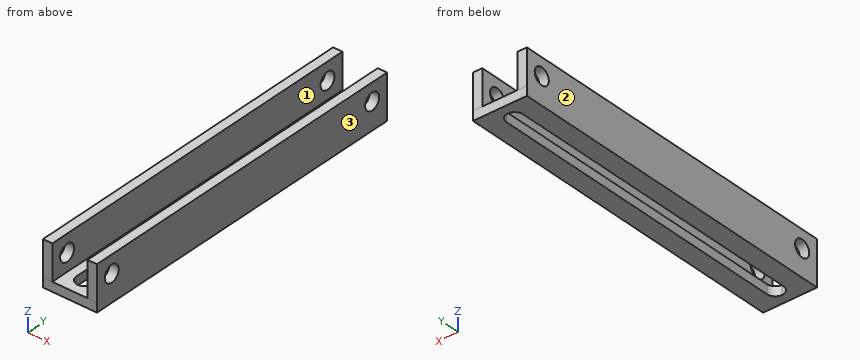
from build123d import *

# Parameters (mm, degrees)
PAD_DEPTH               = 3
SKETCH001_W             = 55.7
SKETCH001_H             = 14.4
SKETCH001_R             = 2.7
PAD001_DEPTH            = 3
PAD_MIRRORED_2_DEPTH    = 3
SKETCH001_MIRRORED_2_W  = 55.7
SKETCH001_MIRRORED_2_H  = 14.4
SKETCH001_MIRRORED_2_R  = 2.7
PAD001_MIRRORED_2_DEPTH = 3


with BuildPart() as part:
    # Sketch → Pad (new body)
    with BuildSketch(Plane.XY):
        with BuildLine():
            ThreePointArc((2.7, 50), (1.909196, 51.909202), (0, 52.700021))
            Line((0, 52.700021), (0, 55.700021))
            Line((0, 55.700021), (8.7, 55.700021))
            Line((8.7, 55.700021), (8.7, 0))
            Line((8.7, 0), (2.7, 0))
            Line((2.7, 0), (2.7, 50))
        make_face()
    pad = extrude(amount=PAD_DEPTH)

    # Sketch001 → Pad001 (join)
    with BuildSketch(Plane.YZ.offset(8.7)):
        with Locations((27.85, 7.2)):
            Rectangle(SKETCH001_W, SKETCH001_H)
        with Locations((50, 8.7)):
            Circle(SKETCH001_R, mode=Mode.SUBTRACT)
    pad001 = extrude(amount=-PAD001_DEPTH)

    # Sketch Mirrored 2 → Pad Mirrored 2 (add)
    with BuildSketch(Plane(origin=(0, 0, 0), x_dir=(-1, 0, 0), z_dir=(0, 0, -1))):
        with BuildLine():
            ThreePointArc((2.7, 50), (1.909196, 51.909202), (0, 52.700021))
            Line((0, 52.700021), (0, 55.700021))
            Line((0, 55.700021), (8.7, 55.700021))
            Line((8.7, 55.700021), (8.7, 0))
            Line((8.7, 0), (2.7, 0))
            Line((2.7, 0), (2.7, 50))
        make_face()
    pad_mirrored_2 = extrude(amount=-PAD_MIRRORED_2_DEPTH)

    # Sketch001 Mirrored 2 → Pad001 Mirrored 2 (add)
    with BuildSketch(Plane.YZ.offset(-8.7)):
        with Locations((27.85, 7.2)):
            Rectangle(SKETCH001_MIRRORED_2_W, SKETCH001_MIRRORED_2_H)
        with Locations((50, 8.7)):
            Circle(SKETCH001_MIRRORED_2_R, mode=Mode.SUBTRACT)
    pad001_mirrored_2 = extrude(amount=PAD001_MIRRORED_2_DEPTH)

    # Mirrored001: Pad, Pad001, Pad Mirrored 2, Pad001 Mirrored 2 across Sketch H_Axis
    add(pad.mirror(Plane.ZX))
    add(pad001.mirror(Plane.ZX))
    add(pad_mirrored_2.mirror(Plane.ZX))
    add(pad001_mirrored_2.mirror(Plane.ZX))


solid = part.part
The model under review builds one solid part; all positions refer to its coordinate system, in mm. Face numbers are marked on the shaded views. Round coordinates to 2 decimals unless told otherwise and drop trailing zeros. Loops run counter-clockwise (first coordinate to the right, second up) from the corner with the lowest first, then second, coordinate; pieces in that order, holes last. Notation, with made-up numbers: (-10.5, 40.5) -> (18.5, 40.5) arc R28 cw to (18.5, 64.5) -> close; hole circle Ø7 at (-23, 5). An arc over 180 degrees is marked (long way). One line per question, with ' | ' between items. Start each with the question number.
Item 1: Draft analysis for pull direction X (two halves, no side actions). For the marked faces 1, 2 and 3, state which applies: +X half, -X half, draft (parallel to the pull), parting line (faces both ways), or undercut.
Item 2: Wall thickness on line 1 along Z through (x, y) = (6.65, 50); line 2 along X through (y, z) = (-16, 5); line 3 along Y through (x, z) = (-6.25, 11): over which ranges is each line inside the solid? List them lowest first. Write a range as [from, to].
Item 3: Add section A-A, the plane z = 8.7. Write out the cut boundary in (x, y), then the cut area to 3 significant figures.
Item 4: Add section B-B, the plane y = -8.5. Write out the cut boundary in (x, z).
Item 5: Add section C-C, the plane x = 1.25. Write out the cut boundary in (y, z).
Return value:
1) face 1: undercut | face 2: -X half | face 3: +X half
2) line 1: z = [0, 6], [11.4, 14.4] | line 2: x = [-8.7, -5.7], [5.7, 8.7] | line 3: y = [-55.7, -51.41], [-48.59, 48.59], [51.41, 55.7]
3) outline: (-8.7, -55.7) -> (-5.7, -55.7) -> (-5.7, -52.7) -> (-8.7, -52.7) -> close; (-8.7, -47.3) -> (-5.7, -47.3) -> (-5.7, 47.3) -> (-8.7, 47.3) -> close; (-8.7, 52.7) -> (-5.7, 52.7) -> (-5.7, 55.7) -> (-8.7, 55.7) -> close; (5.7, -55.7) -> (8.7, -55.7) -> (8.7, -52.7) -> (5.7, -52.7) -> close; (5.7, -47.3) -> (8.7, -47.3) -> (8.7, 47.3) -> (5.7, 47.3) -> close; (5.7, 52.7) -> (8.7, 52.7) -> (8.7, 55.7) -> (5.7, 55.7) -> close | area: 604 mm2
4) outline: (-8.7, 0) -> (-2.7, 0) -> (-2.7, 3) -> (-5.7, 3) -> (-5.7, 14.4) -> (-8.7, 14.4) -> close; (2.7, 0) -> (8.7, 0) -> (8.7, 14.4) -> (5.7, 14.4) -> (5.7, 3) -> (2.7, 3) -> close
5) outline: (-55.7, 0) -> (-52.39, 0) -> (-52.39, 3) -> (-55.7, 3) -> close; (52.39, 0) -> (55.7, 0) -> (55.7, 3) -> (52.39, 3) -> close
